Geometry: final body of the model. Coordinates: model frame, mm. A direction names the side the tool comes from. Coordinates: 2 decimals unless noted, no trailing zeros. Loops run counter-clockwise (first coordinate to the right, second up) from the corner with the lowest first, then second, coordinate; pieces in that order, holes last. Notation, with made-up numbers: (18, -6) - (49, -6) arc R18 cw to (49, 20) - close; hole circle Ø2 at (20.25, 72). An arc over 180 degrees is marked (long way). Put each result on its own line as item: value. Start each with the question number.
1) Material intervals for line 1 along X through (y, z) = (2.5, 9.5); line 2 along X through (y, z) = (-3, 3.25), sorted ascending. Write a range as from..to.
2) Contact query for flat-ended pins moving along their axis: pin 1 Ø8 at (y, z) = (-8, 9.5) entering from +X; pin 2 Ø4 at (y, z) = (-7, 9) entering from +X; pin 3 Ø1.1 at (x, y) = (110, -6) entering from -Z. Output: stop coordinate, or through.
3) Section A-A on y = -2. Output: boundary loops of the cut face in (x, z).
4) Reachability of faces 1 (the flat face through (109, 0, 3.81)), 2 (the flat face through (57, 0, 13.97)) from +Z, -Z, +X, -X, +Y, -Y: full face, straight path, thin tool, end or side. Return the list, or none.
5) Section B-B on z = 7.75. Output: boundary loops of the cut face in (x, y) (3 decimals), and give its area (3 significant figures).
6) Section C-C on z = 1.5. Output: boundary loops of the cut face in (x, y) (3 decimals).
```python
from build123d import *

# Parameters (mm, degrees)
F1_DEPTH = 15.875


with BuildPart() as f1:
    # F0 (on Front) → F1 (new body, symmetric)
    with BuildSketch(Plane.XZ):
        Polygon((107.454668, 3.81), (0, 0), (106.502168, 0), align=None)
        Polygon((-0.495332, 13.97), (0, 0), (107.454668, 3.81), (111.264668, 3.81), (113.804668, 13.97), align=None)
    extrude(amount=F1_DEPTH, both=True)


solid = f1.part
```
Answer block:
1. line 1: x = -0.34..112.69
1. line 2: x = -0.12..107.31
2. pin 1: stops at x = 113.69
2. pin 2: stops at x = 113.06
2. pin 3: stops at z = 3.81
3. outline: (-0.5, 13.97) - (0, 0) - (106.5, 0) - (107.45, 3.81) - (111.26, 3.81) - (113.8, 13.97) - close
4. face 1: -Z, +X, +Y, -Y
4. face 2: +Z, +X, -X, +Y, -Y
5. outline: (-0.275, -15.875) - (112.25, -15.875) - (112.25, 15.875) - (-0.275, 15.875) - close
5. area: 3,570 mm²
6. outline: (-0.053, -15.875) - (106.877, -15.875) - (106.877, 15.875) - (-0.053, 15.875) - close
